Read the model definition and answer for the solid it produces. Units are mm, in the model's axes. A direction names the side the tool comes from. Give positions to 0.01 mm unless a question says otherwise; leave off trailing zeros. Loops run counter-clockwise (first coordinate to the right, second up) from the corner with the lowest first, then second, coordinate; pieces in that order, holes last.
(1) Find section B-B, the plane x = 25.4. Write down the section's boundary in (y, z) (3 decimals), then the cut area to 3 significant figures.
(2) Find section C-C, the plane z = 9.75. Write down the section's boundary in (x, y) (3 decimals), then the cut area to 3 significant figures.
(3) Which of the six approach directions +Z, -Z, +X, -X, +Y, -Y give full straight-line access (tool end or side, diameter ignored) to faces 5 (the face through (36.574, 14.099, 23.835)), 6 (the face through (63, 3.175, 13))?
(4) Find section A-A, the plane y = 25.4. Write down the section's boundary in (x, z) (1 decimal).
(5) Straight lines are drawn through the part: probe 1 along Z at (x, y) = (40, 34) (3 decimals); probe 2 along Y at (x, z) = (59, 19) (3 decimals); probe 3 along Y at (x, z) = (38.1, 0.7). For each, find the intervals that lie inside material, in ascending order.
(6) Find section D-D, the plane y = 34. Write down the section's boundary in (x, z) (3 decimals).
(7) Determine the mould class of faces 1 (the face through (64, 47.625, 13)), 2 (the face through (12.431, 14.752, 1.61)), 3 (the face through (0, 26, 2)), 4 (the face through (127, 25, 2)) for opening direction X: pulls with the +X half, pulls with the -X half, needs draft (parallel to the pull), parting line crosses it, or undercut.
Autodesk Inventor part; units mm, degrees
ref_plane "YZ Plane" through (0, 0, 0) normal (1, 0, 0) x (0, 1, 0)
ref_plane "XZ Plane" through (0, 0, 0) normal (0, 1, 0) x (-1, 0, 0)
ref_plane "XY Plane" through (0, 0, 0) normal (0, 0, 1) x (1, 0, 0)
sketch "Sketch1" plane through (0, 0, 0) normal (0, 0, 1) x (1, 0, 0)
  line L0 (0, 0) -> (127, 0)
  line L1 (127, 0) -> (127, 50.8)
  line L2 (127, 50.8) -> (0, 50.8)
  line L3 (0, 50.8) -> (0, 0)
  dimension "d0" = 50.8
  dimension "d1" = 127
extrude "Extrusion1" add sketch "Sketch1" along normal blind 25.4
shell "Shell1" thickness 3.175 removed faces 2 at (0, 33.8667, 16.9333) at (127, 16.9333, 8.4667)
sketch "Sketch2" plane through (0, 0, 25.4) normal (0, 0, 1) x (1, 0, 0)
  line L0 (0, 3.175) -> (0, 47.625)
  line L1 (0, 25.4) -> (101.6, 25.4)
  circle A0 centre (101.6, 25.4) radius 14.2875
  line L2 (127, 0) -> (127, 50.8)
  point P0 (0, 0)
  dimension "d5" = 28.575
  dimension "d9" = 25.4
extrude "Extrusion2" cut sketch "Sketch2" against normal through all
sketch "Sketch3" plane through (0, 0, 25.4) normal (0, 0, 1) x (1, 0, 0)
  line L0 (0, 50.8) -> (0, 12.7)
  line L1 (0, 3.175) -> (0, 47.625)
  line L2 (0, 12.7) -> (12.7, 12.7)
  circle A0 centre (12.7, 12.7) radius 2.0701
  circle A1 centre (25.4, 12.7) radius 2.0701
  circle A2 centre (38.1, 12.7) radius 2.0701
  point P0 (0, 0)
  dimension "d12" = 12.7
  dimension "d13" = 4.1402
  dimension "d16" = 12.7
  dimension "d23" = 12.7
extrude "Extrusion3" cut sketch "Sketch3" against normal through all
properties part number "Intake mount"
Entries:
1. outline: (0, 0) - (10.63, 0) - (10.63, 3.175) - (3.175, 3.175) - (3.175, 22.225) - (10.63, 22.225) - (10.63, 25.4) - (0, 25.4) - close; (14.77, 0) - (50.8, 0) - (50.8, 25.4) - (14.77, 25.4) - (14.77, 22.225) - (47.625, 22.225) - (47.625, 3.175) - (14.77, 3.175) - close
1. area: 417 mm2
2. outline: (0, 0) - (127, 0) - (127, 3.175) - (0, 3.175) - close; (0, 47.625) - (127, 47.625) - (127, 50.8) - (0, 50.8) - close
2. area: 806 mm2
3. face 5: +Z, -Z
3. face 6: +X, -X
4. outline: (0, 0) - (87.3, 0) - (87.3, 3.2) - (0, 3.2) - close; (0, 22.2) - (87.3, 22.2) - (87.3, 25.4) - (0, 25.4) - close; (115.9, 0) - (127, 0) - (127, 3.2) - (115.9, 3.2) - close; (115.9, 22.2) - (127, 22.2) - (127, 25.4) - (115.9, 25.4) - close
5. probe 1: z = 0 to 3.175, 22.225 to 25.4
5. probe 2: y = 0 to 3.175, 47.625 to 50.8
5. probe 3: y = 0 to 10.63, 14.77 to 50.8
6. outline: (0, 0) - (90.191, 0) - (90.191, 3.175) - (0, 3.175) - close; (0, 22.225) - (90.191, 22.225) - (90.191, 25.4) - (0, 25.4) - close; (113.009, 0) - (127, 0) - (127, 3.175) - (113.009, 3.175) - close; (113.009, 22.225) - (127, 22.225) - (127, 25.4) - (113.009, 25.4) - close
7. face 1: needs draft
7. face 2: undercut
7. face 3: pulls with the -X half
7. face 4: pulls with the +X half
